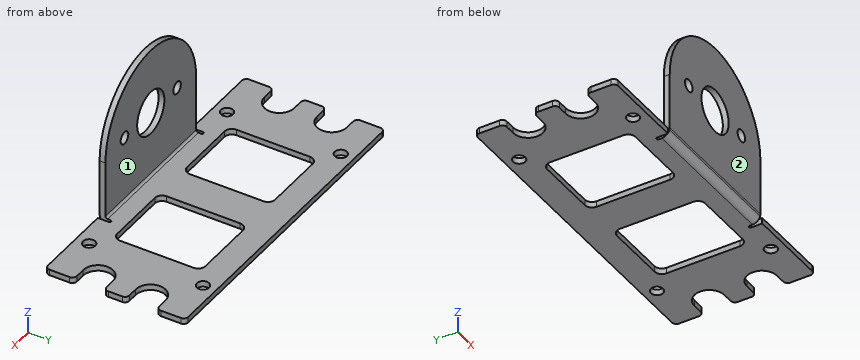
```python
from build123d import *

# Parameters (mm, degrees)
SKETCH1_R                = 2.1
BASE_FLANGE1_DEPTH       = 2
EDGE_FLANGE1_START       = -3
EDGE_FLANGE1_DEPTH       = 3.7366
EDGE_FLANGE1_START_2     = 0.7366
EDGE_FLANGE1_2_OUTLINE_W = 50
EDGE_FLANGE1_2_OUTLINE_H = 2
EDGE_FLANGE1_2_DEPTH     = 44.2634
EDGE_FLANGE1_START_3     = -25
EDGE_FLANGE1_3_DEPTH     = 50
EDGE_FLANGE1_4_DEPTH     = 50
FILLET1_RADIUS           = 25
FILLET1_LENGTH           = 2
CUT_EXTRUDE1_REACH       = 86.652
SKETCH9_R                = 7.5
SKETCH9_R_2              = 2.1


with BuildPart() as part:
    # Base-Flange1: sheet metal written as solids
    # Sketch1 → Base-Flange1 (new body)
    with BuildSketch(Plane.XY):
        with BuildLine():
            Line((-53.5, -24), (53.5, -24))
            ThreePointArc((53.5, -24), (54.560660172, -23.560660172), (55, -22.5))
            Line((55, -22.5), (55, -15.6))
            ThreePointArc((55, -15.6), (54.560660172, -14.539339828), (53.5, -14.1))
            Line((53.5, -14.1), (50, -14.1))
            ThreePointArc((50, -14.1), (44.9, -9), (50, -3.9))
            Line((50, -3.9), (53.5, -3.9))
            ThreePointArc((53.5, -3.9), (54.560660172, -3.460660172), (55, -2.4))
            Line((55, -2.4), (55, 2.4))
            ThreePointArc((55, 2.4), (54.560660172, 3.460660172), (53.5, 3.9))
            Line((53.5, 3.9), (50, 3.9))
            ThreePointArc((50, 3.9), (44.9, 9), (50, 14.1))
            Line((50, 14.1), (53.5, 14.1))
            ThreePointArc((53.5, 14.1), (54.560660172, 14.539339828), (55, 15.6))
            Line((55, 15.6), (55, 22.5))
            ThreePointArc((55, 22.5), (54.560660172, 23.560660172), (53.5, 24))
            Line((53.5, 24), (-53.5, 24))
            ThreePointArc((-53.5, 24), (-54.560660172, 23.560660172), (-55, 22.5))
            Line((-55, 22.5), (-55, 15.6))
            ThreePointArc((-55, 15.6), (-54.560660172, 14.539339828), (-53.5, 14.1))
            Line((-53.5, 14.1), (-50, 14.1))
            ThreePointArc((-50, 14.1), (-44.9, 9), (-50, 3.9))
            Line((-50, 3.9), (-53.5, 3.9))
            ThreePointArc((-53.5, 3.9), (-54.560660172, 3.460660172), (-55, 2.4))
            Line((-55, 2.4), (-55, -2.4))
            ThreePointArc((-55, -2.4), (-54.560660172, -3.460660172), (-53.5, -3.9))
            Line((-53.5, -3.9), (-50, -3.9))
            ThreePointArc((-50, -3.9), (-44.9, -9), (-50, -14.1))
            Line((-50, -14.1), (-53.5, -14.1))
            ThreePointArc((-53.5, -14.1), (-54.560660172, -14.539339828), (-55, -15.6))
            Line((-55, -15.6), (-55, -22.5))
            ThreePointArc((-55, -22.5), (-54.560660172, -23.560660172), (-53.5, -24))
        make_face()
        with Locations((-38, 19.5)):
            Circle(SKETCH1_R, mode=Mode.SUBTRACT)
        with Locations((-38, -19.5)):
            Circle(SKETCH1_R, mode=Mode.SUBTRACT)
        with Locations((38, 19.5)):
            Circle(SKETCH1_R, mode=Mode.SUBTRACT)
        with Locations((38, -19.5)):
            Circle(SKETCH1_R, mode=Mode.SUBTRACT)
        with BuildLine():
            Line((6.4, 12.6), (6.4, -12.6))
            ThreePointArc((6.4, -12.6), (7.132233047, -14.367766953), (8.9, -15.1))
            Line((8.9, -15.1), (29.6, -15.1))
            ThreePointArc((29.6, -15.1), (31.367766953, -14.367766953), (32.1, -12.6))
            Line((32.1, -12.6), (32.1, 12.6))
            ThreePointArc((32.1, 12.6), (31.367766953, 14.367766953), (29.6, 15.1))
            Line((29.6, 15.1), (8.9, 15.1))
            ThreePointArc((8.9, 15.1), (7.132233047, 14.367766953), (6.4, 12.6))
        make_face(mode=Mode.SUBTRACT)
        with BuildLine():
            Line((-6.4, 12.6), (-6.4, -12.6))
            ThreePointArc((-6.4, -12.6), (-7.132233047, -14.367766953), (-8.9, -15.1))
            Line((-8.9, -15.1), (-29.6, -15.1))
            ThreePointArc((-29.6, -15.1), (-31.367766953, -14.367766953), (-32.1, -12.6))
            Line((-32.1, -12.6), (-32.1, 12.6))
            ThreePointArc((-32.1, 12.6), (-31.367766953, 14.367766953), (-29.6, 15.1))
            Line((-29.6, 15.1), (-8.9, 15.1))
            ThreePointArc((-8.9, 15.1), (-7.132233047, 14.367766953), (-6.4, 12.6))
        make_face(mode=Mode.SUBTRACT)
    extrude(amount=-BASE_FLANGE1_DEPTH)

    # Edge-Flange1: read off the stored shape, not the designer's step
    # Edge-Flange1 outline → Edge-Flange1 (cut)
    with BuildSketch(Plane.XY.offset(EDGE_FLANGE1_START)):
        with BuildLine():
            Line((-26, -24), (-25, -24))
            Line((-25, -24), (-25, -20.2634))
            ThreePointArc((-25, -20.2634), (-25.5, -19.7634), (-26, -20.2634))
            Line((-26, -20.2634), (-26, -24))
        make_face()
        with BuildLine():
            Line((25, -20.2634), (25, -24))
            Line((25, -24), (26, -24))
            Line((26, -24), (26, -20.2634))
            ThreePointArc((26, -20.2634), (25.5, -19.7634), (25, -20.2634))
        make_face()
    extrude(amount=EDGE_FLANGE1_DEPTH, mode=Mode.SUBTRACT)

    # Edge-Flange1 3 outline → Edge-Flange1 3 (cut)
    with BuildSketch(Plane.YZ.offset(EDGE_FLANGE1_START_3)):
        with BuildLine():
            ThreePointArc((-21.2634, -2), (-22.917667209, -1.443395312), (-23.899002398, 0))
            Line((-23.899002398, 0), (-24, 0))
            Line((-24, 0), (-24, -2))
            Line((-24, -2), (-21.2634, -2))
        make_face()
    extrude(amount=EDGE_FLANGE1_3_DEPTH, mode=Mode.SUBTRACT)



with BuildPart() as body_2:
    # Edge-Flange1 2 outline → Edge-Flange1 2 (new body)
    with BuildSketch(Plane.XY.offset(EDGE_FLANGE1_START_2)):
        with Locations((0, -23)):
            Rectangle(EDGE_FLANGE1_2_OUTLINE_W, EDGE_FLANGE1_2_OUTLINE_H)
    extrude(amount=EDGE_FLANGE1_2_DEPTH)


with BuildPart() as part_1:
    add(part.part)

    add(body_2.part)  # Edge-Flange1 4 merges body 2
    # Edge-Flange1 4 outline → Edge-Flange1 4 (add)
    with BuildSketch(Plane.YZ.offset(EDGE_FLANGE1_START_3)):
        with BuildLine():
            Line((-22, 0.7366), (-24, 0.7366))
            ThreePointArc((-24, 0.7366), (-23.974633029, 0.364854094), (-23.899002398, 0))
            Line((-23.899002398, 0), (-21.2634, 0))
            ThreePointArc((-21.2634, 0), (-21.784254855, 0.215745145), (-22, 0.7366))
        make_face()
    extrude(amount=EDGE_FLANGE1_4_DEPTH)

    # Fillet1: full round fillet: the end face becomes a half cylinder, R = half its width
    fillet1_face = Plane((0, -23, 45), x_dir=(0, -1, 0), z_dir=(0, 0, 1))  # on the end face: x along it, z out of the body
    fillet1_slab = fillet1_face.offset(-FILLET1_RADIUS / 2) * Box(FILLET1_LENGTH, 2 * FILLET1_RADIUS, FILLET1_RADIUS, mode=Mode.PRIVATE)  # the body's end, R deep
    fillet1_round = Plane((0, -23, 20), x_dir=(0, 0, 1), z_dir=(0, -1, 0)) * Cylinder(FILLET1_RADIUS, FILLET1_LENGTH, mode=Mode.PRIVATE)  # its axis R under the face
    add(fillet1_slab - fillet1_round, mode=Mode.SUBTRACT)

    # Sketch9 → Cut-Extrude1 (cut, up to next)
    with BuildSketch(Plane(origin=(0, -22, 0), x_dir=(1, 0, 0), z_dir=(0, 1, 0)), mode=Mode.PRIVATE) as cut_extrude1_sk1:
        with Locations(Location((0, -22.5, 0), (0, 0, 180))):
            Circle(SKETCH9_R)
    cut_extrude1_tool1 = extrude(cut_extrude1_sk1.sketch, amount=-CUT_EXTRUDE1_REACH, mode=Mode.PRIVATE) & part_1.part
    # Sketch9 → Cut-Extrude1 (cut, up to next)
    with BuildSketch(Plane(origin=(0, -22, 0), x_dir=(1, 0, 0), z_dir=(0, 1, 0)), mode=Mode.PRIVATE) as cut_extrude1_sk2:
        with Locations(Location((-14.5, -22.5, 0), (0, 0, 180))):
            Circle(SKETCH9_R_2)
    cut_extrude1_tool2 = extrude(cut_extrude1_sk2.sketch, amount=-CUT_EXTRUDE1_REACH, mode=Mode.PRIVATE) & part_1.part
    # Sketch9 → Cut-Extrude1 (cut, up to next)
    with BuildSketch(Plane(origin=(0, -22, 0), x_dir=(1, 0, 0), z_dir=(0, 1, 0)), mode=Mode.PRIVATE) as cut_extrude1_sk3:
        with Locations(Location((14.5, -22.5, 0), (0, 0, 180))):
            Circle(SKETCH9_R_2)
    cut_extrude1_tool3 = extrude(cut_extrude1_sk3.sketch, amount=-CUT_EXTRUDE1_REACH, mode=Mode.PRIVATE) & part_1.part
    add(cut_extrude1_tool1.solids().sort_by_distance((0, -22, 22.5))[0], mode=Mode.SUBTRACT)
    add(cut_extrude1_tool2.solids().sort_by_distance((-14.5, -22, 22.5))[0], mode=Mode.SUBTRACT)
    add(cut_extrude1_tool3.solids().sort_by_distance((14.5, -22, 22.5))[0], mode=Mode.SUBTRACT)


solid = part_1.part
```
Can you work these out from the model? Positions are in its coordinate system, mm. Face numbers are marked on the shaded views. A direction names the side the tool comes from. Coordinates: 2 decimals unless noted, no trailing zeros. Loops run counter-clockwise (first coordinate to the right, second up) from the corner with the lowest first, then second, coordinate; pieces in that order, holes last. Notation, with made-up numbers: (-25, 72) - (-2, 72) arc R37 ccw to (-2, 109) - close; hole circle Ø9 at (-13.75, 1). An arc over 180 degrees is marked (long way). Use a Markdown table: item, result.
Item 1: I want a section at A-A on y = -9. Please give me the cut outline in (x, z), and give its area (3 significant figures).
Numbers:
| item | result |
|---|---|
| outline | (-44.9, -2) - (-32.1, -2) - (-32.1, 0) - (-44.9, 0) - close; (-6.4, -2) - (6.4, -2) - (6.4, 0) - (-6.4, 0) - close; (32.1, -2) - (44.9, -2) - (44.9, 0) - (32.1, 0) - close |
| area | 76.8 mm2 |
Item 2: I want a section at D-D on x = -14.5. Please give me the cut outline in (y, z), and give its area (3 significant figures).
Numbers:
| item | result |
|---|---|
| outline | (-24, 0.74) arc R2.74 ccw to (-21.26, -2) - (-15.1, -2) - (-15.1, 0) - (-21.26, 0) arc R0.74 cw to (-22, 0.74) - (-22, 20.4) - (-24, 20.4) - close; (-24, 24.6) - (-22, 24.6) - (-22, 40.37) - (-24, 40.37) - close; (15.1, -2) - (24, -2) - (24, 0) - (15.1, 0) - close |
| area | 106 mm2 |
Item 3: For the marked faces 1 and 2, which set-ups out of +Z, -Z, +X, -X, +Y, -Y let a thin tool reach every point of the face, with its end or its side?
Numbers:
| item | result |
|---|---|
| face 1 | +Z, +X, -X, +Y |
| face 2 | +Z, -Z, +X, -X, -Y |
Item 4: Will these pins go through, and if not, where does the flat tip stop? pin 1 (1.1 mm diameter, centred on y = -23, z = 12, fed in from -X); pin 2 (0.6 mm diameter, centred on x = 22.5, z = -1.5, fed in from -Y); pin 3 (3 mm diameter, centred on y = -22.5, z = 11, fed in from +X).
Numbers:
| item | result |
|---|---|
| pin 1 | stops at x = -25 |
| pin 2 | stops at y = -23.2 |
| pin 3 | stops at x = 25 |
Item 5: I want a section at B-B on x = 0. Please give me the cut outline in (y, z), and give its area (3 significant figures).
Numbers:
| item | result |
|---|---|
| outline | (-24, 0.74) arc R2.74 ccw to (-21.26, -2) - (24, -2) - (24, 0) - (-21.26, 0) arc R0.74 cw to (-22, 0.74) - (-22, 15) - (-24, 15) - close; (-24, 30) - (-22, 30) - (-22, 45) - (-24, 45) - close |
| area | 155 mm2 |
Item 6: If I drill on probe 1 along Y at (x, z) = (-38, -1.2); probe 2 along Z at (x, y) = (-41, -14); probe 3 along X at (y, z) = (-23, 22), over which ranges is the centre line in solid material (lowest first)? Write a range as from..to.
Numbers:
| item | result |
|---|---|
| probe 1 | y = -24..-21.6, -17.4..17.4, 21.6..24 |
| probe 2 | z = -2..0 |
| probe 3 | x = -24.92..-16.54, -12.46..-7.48, 7.48..12.46, 16.54..24.92 |
Item 7: I want a section at C-C on z = 22.5. Please give me the cut outline in (x, y), and give its area (3 significant figures).
Numbers:
| item | result |
|---|---|
| outline | (-24.87, -24) - (-16.6, -24) - (-16.6, -22) - (-24.87, -22) - close; (-12.4, -24) - (-7.5, -24) - (-7.5, -22) - (-12.4, -22) - close; (7.5, -24) - (12.4, -24) - (12.4, -22) - (7.5, -22) - close; (16.6, -24) - (24.87, -24) - (24.87, -22) - (16.6, -22) - close |
| area | 52.7 mm2 |
